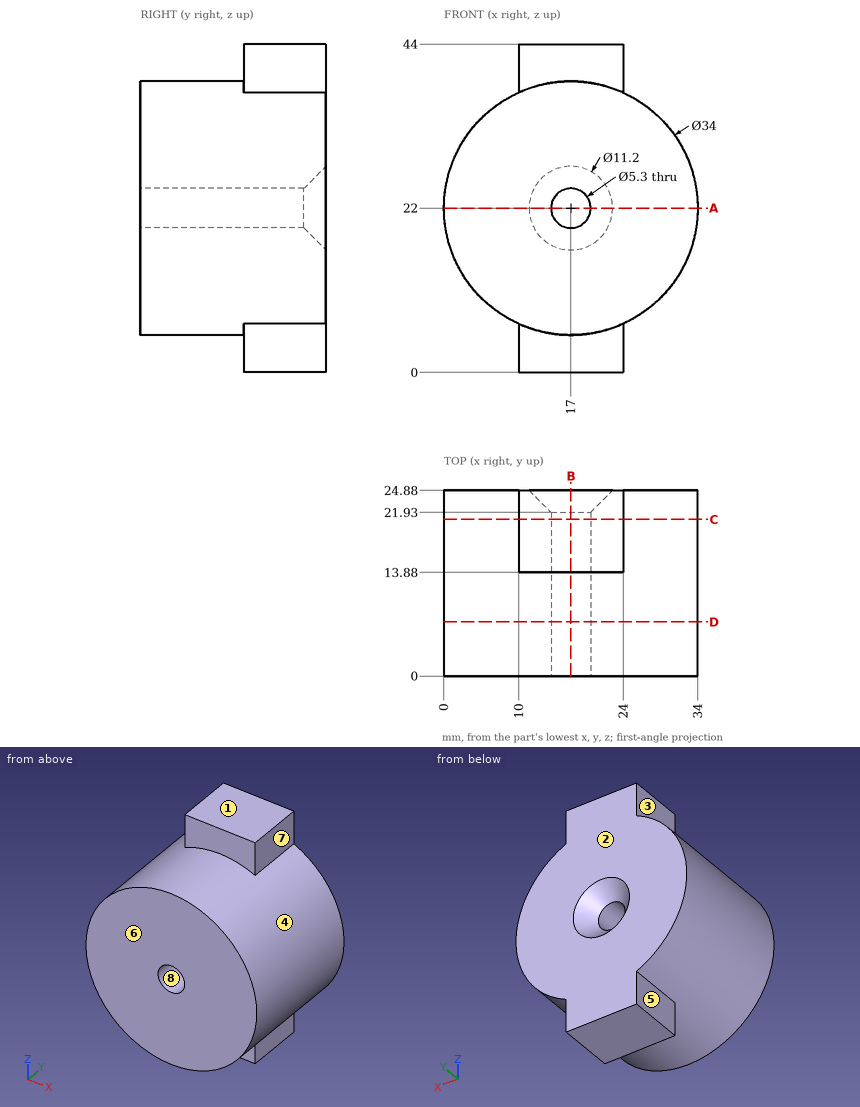
Answer from the drawing. Dimensions are ordinates in mm from the lowest x, y and z of the part. A direction names the side the tool comes from. Round coordinates to 2 decimals unless told otherwise and drop trailing zeros. Write each loop counter-clockwise with the first axis right and the second up, starting at its lowest first coordinate (ties: lowest second). Pieces come first, ordered by that corner, then holes. Notation, with made-up numbers: (63, -19) - (97, -19) arc R22 ccw to (97, -8) - close; hole circle Ø6 at (24, 56.25). An arc over 180 degrees is marked (long way). One line per item, written item: value.
Q1. Each of these flat-tipped pins is pushed along its axis until it touches: P1, Ø2, axis at x = 20, z = 41.5, coming from the -Y side; P2, Ø12, axis at x = 23, y = 5, coming from the +Z side; P3, Ø1, axis at y = 3.5, z = 19.5, coming from the -X side. Where does it stop, or does it pass through?
The answers:
P1: stops at y = 13.88
P2: stops at z = 39
P3: stops at x = 0.12
Q2. Find section D-D (y = 7.25). Determine the outline of the cut face in (x, z), and give its area (3 significant figures).
The answers:
outline: circle Ø34 at (17, 22); hole circle Ø5.3 at (17, 22)
area: 886 mm2
Q3. Which of the six approach directions +Z, -Z, +X, -X, +Y, -Y give full straight-line access (tool end or side, diameter ignored) to the marked faces 1, 2, 3, 4 and 5?
The answers:
face 1: +Z, +X, -X, +Y, -Y
face 2: +Z, -Z, +X, -X, +Y
face 3: +Z, -X, +Y, -Y
face 4: -Y
face 5: -Z, -X, +Y, -Y
Q4. Find section B-B (x = 17). Determine the outline of the cut face in (y, z).
The answers:
outline: (0, 5) - (13.88, 5) - (13.88, 0) - (24.88, 0) - (24.88, 16.4) - (21.93, 19.35) - (0, 19.35) - close; (0, 24.65) - (21.93, 24.65) - (24.88, 27.6) - (24.88, 44) - (13.88, 44) - (13.88, 39) - (0, 39) - close
Q5. Find section A-A (z = 22). Determine the outline of the cut face in (x, y), and give its area (3 significant figures).
The answers:
outline: (0, 0) - (14.35, 0) - (14.35, 21.93) - (11.4, 24.88) - (0, 24.88) - close; (19.65, 0) - (34, 0) - (34, 24.88) - (22.6, 24.88) - (19.65, 21.93) - close
area: 705 mm2
Q6. For a pull along X with two mould halves and no side action, classify the marked faces 6, 7 and 8 as pulls with the +X half, pulls with the -X half, needs draft (parallel to the pull), parting line crosses it, or undercut.
The answers:
face 6: needs draft
face 7: pulls with the +X half
face 8: undercut
Q7. Straight lines are drawn through the part: line 1 (X direction, y = 10.5, z = 22); line 2 (Z direction, x = 17, y = 9.5); line 3 (Z direction, x = 17, y = 15.5). For each, find the intervals that lie inside material, in ascending order. Write a range as from..to.
The answers:
line 1: x = 0..14.35, 19.65..34
line 2: z = 5..19.35, 24.65..39
line 3: z = 0..19.35, 24.65..44
Q8. Find section C-C (y = 21). Determine the outline of the cut face in (x, z), and give its area (3 significant figures).
The answers:
outline: (10, 0) - (24, 0) - (24, 6.51) arc R17 ccw to (24, 37.49) - (24, 44) - (10, 44) - (10, 37.49) arc R17 ccw to (10, 6.51) - close; hole circle Ø5.3 at (17, 22)
area: 1,040 mm2
